```python
from build123d import *

# Parameters (mm, degrees)
SKETCH_335_R           = 15
EXTRUDE_380_DEPTH      = 10
EXTRUDE_START          = -2.5
EXTRUDE_822_DEPTH      = 9.5
SKETCH_883_R           = 9.65
CUT_EXTRUDE_1089_DEPTH = 8.5
SKETCH_4_3_R           = 11.15
SKETCH_4_3_R_2         = 9.65
CUT_EXTRUDE_1131_DEPTH = 7
CUT_EXTRUDE_1399_REACH = 66.699
SKETCH_1242_R          = 3.6
EXTRUDE_START_2        = -4
EXTRUDE_3_OUTLINE_R    = 11.15
EXTRUDE_3_DEPTH        = 4
SKETCH_4_5_R           = 14.6
SKETCH_4_5_R_2         = 6.75
SKETCH_4_5_R_3         = 5.25
CUT_EXTRUDE_1_DEPTH    = 3.5


# Read off the part's stored shape, not the designer's step: the extrude step
with BuildPart() as part:
    # Sketch 335 → Extrude 380 (new body)
    with BuildSketch(Plane.XY):
        Circle(SKETCH_335_R)
    extrude(amount=EXTRUDE_380_DEPTH)

    # Sketch 2 → Extrude 822 (add)
    with BuildSketch(Plane(origin=(0, -15, 0), x_dir=(-1, 0, 0), z_dir=(0, -1, 0)).offset(EXTRUDE_START)):
        with BuildLine():
            Line((15, -30), (15, 0))
            Line((15, 0), (-15, 0))
            Line((-15, 0), (-15, -30))
            ThreePointArc((-15, -30), (0, -45), (15, -30))
        make_face()
    extrude_822 = extrude(amount=EXTRUDE_822_DEPTH)

    # Sketch 883 → Cut-Extrude 1089 (cut)
    with BuildSketch(Plane(origin=(0, -12.5, 0), x_dir=(1, 0, 0), z_dir=(0, 1, 0))):
        with Locations(Location((0, -30, 0), (0, 0, 270))):
            Circle(SKETCH_883_R)
    cut_extrude_1089 = extrude(amount=-CUT_EXTRUDE_1089_DEPTH, mode=Mode.SUBTRACT)

    # Sketch 4_3 → Cut-Extrude 1131 (cut)
    with BuildSketch(Plane(origin=(0, -12.5, 0), x_dir=(1, 0, 0), z_dir=(0, 1, 0))):
        with Locations(Location((0, -30, 0), (0, 0, 270))):
            Circle(SKETCH_4_3_R)
        with Locations(Location((0, -30, 0), (0, 0, 270))):
            Circle(SKETCH_4_3_R_2, mode=Mode.SUBTRACT)
    cut_extrude_1131 = extrude(amount=-CUT_EXTRUDE_1131_DEPTH, mode=Mode.SUBTRACT)

    # Mirror 2: Extrude 822, Cut-Extrude 1089, Cut-Extrude 1131 across plane
    add(extrude_822.mirror(Plane.ZX))
    add(cut_extrude_1089.mirror(Plane.ZX), mode=Mode.SUBTRACT)
    add(cut_extrude_1131.mirror(Plane.ZX), mode=Mode.SUBTRACT)

    # Sketch 1242 → Cut-Extrude 1399 (cut, up to next)
    with BuildSketch(Plane(origin=(0, 22, 0), x_dir=(1, 0, 0), z_dir=(0, 1, 0)), mode=Mode.PRIVATE) as cut_extrude_1399_sk1:
        with Locations(Location((0, -30, 0), (0, 0, 270))):
            Circle(SKETCH_1242_R)
    cut_extrude_1399_tool1 = extrude(cut_extrude_1399_sk1.sketch, amount=-CUT_EXTRUDE_1399_REACH, mode=Mode.PRIVATE) & part.part
    add(cut_extrude_1399_tool1.solids().sort_by_distance((0, 22, 30))[0], mode=Mode.SUBTRACT)

    # Extrude 3 outline → Extrude 3 (add)
    with BuildSketch(Plane(origin=(0, 22, 0), x_dir=(1, 0, 0), z_dir=(0, 1, 0)).offset(EXTRUDE_START_2)):
        with BuildLine():
            ThreePointArc((-22.804910758, -26.319504748), (-26.411442066, -35.943355833), (-16.921921975, -39.889820861))
            ThreePointArc((-16.921921975, -39.889820861), (11.293799089, -46.019054345), (15, -17.38413697))
            Line((15, -17.38413697), (15, -30))
            ThreePointArc((15, -30), (0, -45), (-15, -30))
            Line((-15, -30), (-15, -12.432700834))
            ThreePointArc((-15, -12.432700834), (-20.137369493, -18.682034198), (-22.804910758, -26.319504748))
        make_face()
        with Locations((0, -30)):
            Circle(EXTRUDE_3_OUTLINE_R)
    extrude(amount=EXTRUDE_3_DEPTH)

    # Sketch 4_5 → Cut-Extrude 1 (cut)
    # profile 1 of 5: a face of its own
    with BuildSketch(Plane(origin=(0, 22, 0), x_dir=(1, 0, 0), z_dir=(0, 1, 0))):
        with BuildLine():
            ThreePointArc((-15, -30), (0, -45), (15, -30))
            ThreePointArc((15, -30), (0, -15), (-15, -30))
        make_face()
        with Locations(Location((0, -30, 0), (0, 0, 270))):
            Circle(SKETCH_4_5_R, mode=Mode.SUBTRACT)
    # profile 2 of 5: a face of its own
    with BuildSketch(Plane(origin=(0, 22, 0), x_dir=(1, 0, 0), z_dir=(0, 1, 0))):
        with BuildLine():
            ThreePointArc((15.6, -30), (15.449271828, -27.836669235), (15, -25.715142943))
            Line((15, -25.715142943), (15, -30))
            ThreePointArc((15, -30), (0, -45), (-15, -30))
            Line((-15, -30), (-15, -25.715142943))
            ThreePointArc((-15, -25.715142943), (-2.163330765, -45.449271828), (15.6, -30))
        make_face()
    # profile 3 of 5: a face of its own
    with BuildSketch(Plane(origin=(0, 22, 0), x_dir=(1, 0, 0), z_dir=(0, 1, 0))):
        with BuildLine():
            ThreePointArc((15.6, -30), (15.449271828, -27.836669235), (15, -25.715142943))
            Line((15, -25.715142943), (15, -30))
            ThreePointArc((15, -30), (0, -45), (-15, -30))
            Line((-15, -30), (-15, -25.715142943))
            ThreePointArc((-15, -25.715142943), (-2.163330765, -45.449271828), (15.6, -30))
        make_face()
    # profile 4 of 5: a face of its own
    with BuildSketch(Plane(origin=(0, 22, 0), x_dir=(1, 0, 0), z_dir=(0, 1, 0))):
        with BuildLine():
            Line((15, -30), (15, -25.715142943))
            ThreePointArc((15, -25.715142943), (0, -14.4), (-15, -25.715142943))
            Line((-15, -25.715142943), (-15, -30))
            ThreePointArc((-15, -30), (0, -15), (15, -30))
        make_face()
    # profile 5 of 5: a face of its own
    with BuildSketch(Plane(origin=(0, 22, 0), x_dir=(1, 0, 0), z_dir=(0, 1, 0))):
        with Locations(Location((0, -30, 0), (0, 0, 270))):
            Circle(SKETCH_4_5_R_2)
        with Locations(Location((0, -30, 0), (0, 0, 270))):
            Circle(SKETCH_4_5_R_3, mode=Mode.SUBTRACT)
    extrude(amount=-CUT_EXTRUDE_1_DEPTH, mode=Mode.SUBTRACT)


solid = part.part
```
Can you work these out from the model? Positions are in its coordinate system, mm. A direction names the side the tool comes from. Round coordinates to 2 decimals unless told otherwise and drop trailing zeros. Loops run counter-clockwise (first coordinate to the right, second up) from the corner with the lowest first, then second, coordinate; pieces in that order, holes last. Notation, with made-up numbers: M -21,58.25 L 20,58.25 A21 cw 20,90.25 Z; hole C 1.5,71.5 d3. An arc over 180 degrees is marked long. Write item = value, one per line. Start each with the question number.
(1) If we mould it in two halves opening along X, with no side actions, what happens to faces 1 (the face through (0, 22, 30)), 2 (the face through (0, -21, 30)), 3 (the face through (2.899, -20.24, 39.204)), 4 (the face through (0, -17, 45))? For each: released by +X, released by -X, zero draft, split by the parting line, or undercut.
(2) I need wall thicknesses on line 1 along Y through (x, z) = (-5.5, 13.5); line 2 along Y through (x, z) = (4.5, 24); line 3 along X through (y, z) = (19.35, 30). Which ranges of each line are inside material? Lowest first, please.
(3) I'm going to push flat-ended pins straight in: P1, Ø20, axis at x = 0, y = -2, coming from the +Z side; P2, Ø10.5, axis at y = -17, z = 11.5, coming from the -X side; P3, Ø10, axis at x = -3, y = -9.5, coming from the +Z side. Where does each tip first touch, or does it pass through?
(4) Suppose I cut it at B-B on x = 12. Write out the boundary of the cut face in (y, z).
(5) Suppose I cut it at D-D on z = 9. Write out the boundary of the cut face in (x, y), plus the area to 3 significant figures.
(6) Suppose I cut it at A-A on y = -15. Write out the boundary of the cut face in (x, z), plus the area to 3 significant figures.
(7) Which directions (+Z, -Z, +X, -X, +Y, -Y) give clear straight access to the entire face, cutting with the end or side of a thin tool? Please do faces 5 (the face through (3.349, -15.951, 40.635)), 6 (the face through (-15, 16, 12)), 7 (the face through (0, 0, 10)), 8 (the face through (14, 18.5, 36)), 9 (the face through (0, 15, 45)).
Answer block:
q1.face_1 = zero draft
q1.face_2 = undercut
q1.face_3 = undercut
q1.face_4 = split by the parting line
q2.line_1 = -22 to -12.5, 12.5 to 22
q2.line_2 = -22 to -21, 18 to 22
q2.line_3 = -26.39 to -15.6, -14.6 to -6.75, -5.25 to 5.25, 6.75 to 14.6, 15.6 to 19.6
q3.P1 = 10
q3.P2 = -15
q3.P3 = 45
q4.outline = M -22,0 L -12.5,0 L -12.5,39 L -22,39 Z; M -9,0 L 9,0 L 9,10 L -9,10 Z; M 12.5,0 L 22,0 L 22,20.03 L 18.5,20.03 L 18.5,21.68 L 22,21.68 L 22,38.32 L 18.5,38.32 L 18.5,39.97 L 22,39.97 L 22,45.5 L 18,45.5 L 18,39 L 12.5,39 Z
q5.outline = M -15,-22 L 15,-22 L 15,-12.5 L 8.29,-12.5 A15 ccw 8.29,12.5 L 15,12.5 L 15,22 L -15,22 L -15,12.5 L -8.29,12.5 A15 ccw -8.29,-12.5 L -15,-12.5 Z
q5.area = 1,220 mm²
q6.outline = M -15,0 L 15,0 L 15,30 A15 ccw -15,30 Z; hole C 0,30 d22.3
q6.area = 863 mm²
q7.face_5 = none
q7.face_6 = -Z, -X, -Y
q7.face_7 = +Z, +X, -X
q7.face_8 = +Y
q7.face_9 = +Z, -Y
